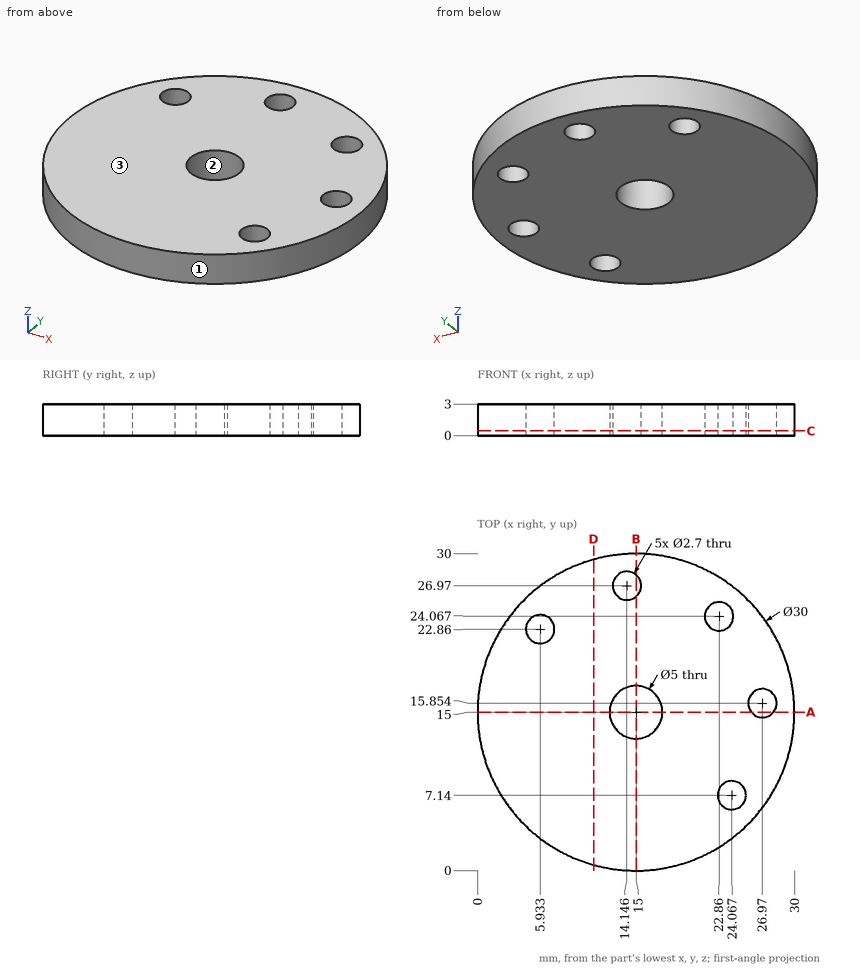
Check sheet for the drawn part. Datum: minimum x, y, z corner. Units: mm. Coordinates: 2 decimals unless noted, no trailing zeros. Write each loop counter-clockwise with the first axis right and the second up, starting at its lowest first coordinate (ties: lowest second). Pieces come first, ordered by that corner, then holes. Notation, with made-up numbers: (38, -39) - (92, -39) arc R21 ccw to (92, -34) - close; hole circle Ø2 at (15, -20). An arc over 180 degrees is marked (long way). Answer as a JSON object with one key per item and string values.
(1) Cross-section at A-A on y = 15. Record the cut outline in (x, z) (1 decimal).
Report:
{"outline": "(0, 0) - (12.5, 0) - (12.5, 3) - (0, 3) - close; (17.5, 0) - (25.9, 0) - (25.9, 3) - (17.5, 3) - close; (28, 0) - (30, 0) - (30, 3) - (28, 3) - close"}
(2) Cross-section at C-C on z = 0.45. Record the cut outline in (x, y).
Report:
{"outline": "circle Ø30 at (15, 15); hole circle Ø2.7 at (5.93, 22.86); hole circle Ø5 at (15, 15); hole circle Ø2.7 at (14.15, 26.97); hole circle Ø2.7 at (22.86, 24.07); hole circle Ø2.7 at (24.07, 7.14); hole circle Ø2.7 at (26.97, 15.85)"}
(3) Cross-section at D-D on x = 11. Record the cut outline in (y, z).
Report:
{"outline": "(0.54, 0) - (29.46, 0) - (29.46, 3) - (0.54, 3) - close"}
(4) Thickness scan on line 1 along Y through (x, z) = (15, 2.25) (1 decimal); line 2 along Y through (x, z) = (14, 2.7); line 3 along X through (y, z) = (24.5, 2.55). Record the ranges inside material, lowest first.
Report:
{"line 1": "0 to 12.5, 17.5 to 25.9, 28 to 30", "line 2": "0.03 to 12.71, 17.29 to 25.63, 28.31 to 29.97", "line 3": "3.39 to 21.58, 24.14 to 26.61"}
(5) Gauge pin test, flat end, axial feed: pin 1 Ø1.6 at (x, y) = (26.97, 15.85) entering from -Z. Record the tip position at first contact, or that the pin passes through.
Report:
{"pin 1": "through"}
(6) Mould release check, pull along X, two halves, no side actions. Record for the marked faces 1, 2 and 3: pulls with the +X half, pulls with the -X half, needs draft (parallel to the pull), parting line crosses it, or undercut.
Report:
{"face 1": "parting line crosses it", "face 2": "undercut", "face 3": "needs draft"}
